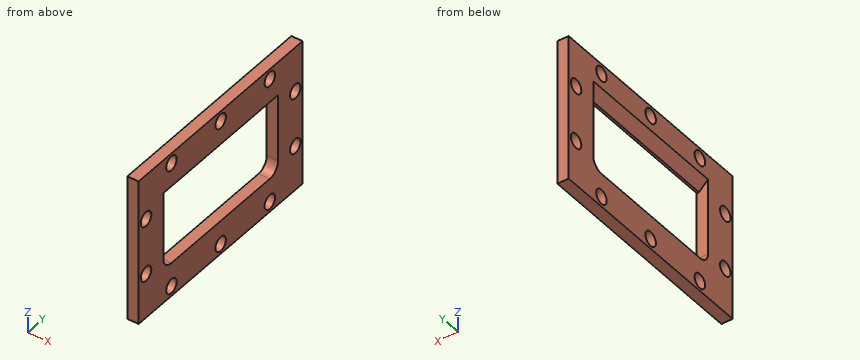
from build123d import *

# Parameters (mm, degrees)
SKETCH1_W           = 99.9998
SKETCH1_H           = 64.99987
BOSS_EXTRUDE1_DEPTH = 4.99999
CUT_EXTRUDE1_DEPTH  = 69.99986
HOLE1_D             = 6.3999872
FILLET1_R           = 4.99999


with BuildPart() as part:
    # Sketch1 → Boss-Extrude1 (new body)
    with BuildSketch(Plane(origin=(0, 0, 0), x_dir=(0, -1, 0), z_dir=(-1, 0, 0))):
        with Locations((-49.9999, 32.499935)):
            Rectangle(SKETCH1_W, SKETCH1_H)
    extrude(amount=-BOSS_EXTRUDE1_DEPTH)

    # Sketch2 → Cut-Extrude1 (cut)
    with BuildSketch(Plane.XZ.offset(-14.99997)):
        Polygon((0, 53.999892), (0, 14.99997), (4.99999, 14.99997), (4.99999, 49.9999), (3.999992, 49.9999), align=None)
    extrude(amount=-CUT_EXTRUDE1_DEPTH, mode=Mode.SUBTRACT)

    # Hole1 (through all)
    with Locations(Plane.ZY):
        with Locations((60.499879, 19.99996), (44.99991, 4.499991), (19.99996, 4.499991), (4.499991, 19.99996), (4.499991, 49.9999), (4.499991, 79.99984), (19.99996, 95.499809), (44.99991, 95.499809), (60.499879, 79.99984), (60.499879, 49.9999)):
            Hole(HOLE1_D / 2)

    # Fillet1
    fillet1_edges = [part.edges().sort_by_distance(p)[0] for p in [
        (2.499995, 84.99983, 14.99997),
        (2.499995, 14.99997, 14.99997),
    ]]
    fillet(fillet1_edges, radius=FILLET1_R)


solid = part.part
Geometry check sheet. Reference: the model listing, model coordinates, mm. Coordinates: 2 decimals unless noted, no trailing zeros. Loops run counter-clockwise (first coordinate to the right, second up) from the corner with the lowest first, then second, coordinate; pieces in that order, holes last. Notation, with made-up numbers: (22, 74.5) - (40, 74.5) arc R6 cw to (40, 82.5) - close; hole circle Ø2 at (7, 89). An arc over 180 degrees is marked (long way). Use one line per item in the form item = value. Start each with the question number.
Item 1: Thickness scan on probe 1 along Y at (x, z) = (3.65, 31.5); probe 2 along Y at (x, z) = (3.6, 5.5); probe 3 along Y at (x, z) = (4.15, 7). Record the ranges inside material, lowest first.
Item 2: Section check B-B, the plane y = 69. Enter the section's corners in (x, z), and give its area (3 significant figures).
Item 3: Section check A-A, the plane z = 38.5. Enter the section's corners in (x, y), and give its area (3 significant figures).
Item 4: Section check D-D, the plane x = 2.1. Give the number of separate pieces and of enclosed holes in the cut face, and give its area (3 significant figures).
Item 5: Section check C-C, the plane z = 59. Enter the section's corners in (x, y), and give its area (3 significant figures).
Item 6: Gauge pin test, flat ends, axial feed: pin 1 (1.5 mm diameter, centred on x = 4, z = 15.5, fed in from -Y); pin 2 (6 mm diameter, centred on y = 4.5, z = 45, fed in from -X). Record the tip position at first contact, or that the pin passes through.
Computed:
q1.probe_1 = 0 to 15, 85 to 100
q1.probe_2 = 0 to 16.96, 23.04 to 46.96, 53.04 to 76.96, 83.04 to 100
q1.probe_3 = 0 to 18, 22 to 48, 52 to 78, 82 to 100
q2.outline = (0, 0) - (5, 0) - (5, 15) - (0, 15) - close; (0, 54) - (4, 50) - (5, 50) - (5, 65) - (0, 65) - close
q2.area = 142 mm2
q3.outline = (0, 0) - (5, 0) - (5, 15) - (0, 15) - close; (0, 85) - (5, 85) - (5, 100) - (0, 100) - close
q3.area = 150 mm2
q4.separate_pieces = 1
q4.enclosed_holes = 11
q4.area = 3,610 mm2
q5.outline = (0, 0) - (5, 0) - (5, 17.17) - (0, 17.17) - close; (0, 22.83) - (5, 22.83) - (5, 47.17) - (0, 47.17) - close; (0, 52.83) - (5, 52.83) - (5, 77.17) - (0, 77.17) - close; (0, 82.83) - (5, 82.83) - (5, 100) - (0, 100) - close
q5.area = 415 mm2
q6.pin_1 = 0
q6.pin_2 = through
